Autodesk Inventor part; units mm, degrees
ref_plane "Work Plane1" through (0, 25, 0) normal (0, 1, 0) x (1, 0, 0)
ref_plane "Work Plane2" through (0, 0, 65) normal (0, 0, -1) x (-1, 0, 0)
ref_plane "YZ Plane" through (0, 0, 0) normal (1, 0, 0) x (0, 1, 0)
sketch "Sketch1" plane through (0, 0, 0) normal (0, 1, 0) x (-1, 0, 0)
  line L0 (0, 0) -> (100, 0)
  line L1 (100, 0) -> (100, 130)
  line L2 (100, 130) -> (0, 130)
  line L3 (0, 130) -> (0, 0)
  dimension "d0" = 130
  dimension "d1" = 100
extrude "Extrusion1" add sketch "Sketch1" along normal blind 50
sketch "Sketch2" plane through (0, 50, 0) normal (0, 1, 0) x (1, 0, 0)
  line L0 (-47, -106) -> (-10, -106)
  line L1 (-10, -106) -> (-10, -24)
  line L2 (-10, -24) -> (-47, -24)
  line L3 (-47, -24) -> (-47, -106)
  line L4 (0, -130) -> (0, 0)
  line L5 (-100, 0) -> (-100, -130)
  line L6 (-100, -130) -> (0, -130)
  line L7 (0, -130) -> (0, 0)
  line L8 (0, 0) -> (-100, 0)
  line L9 (-100, -65) -> (0, -65) construction
  point P0 (-47, -65)
  dimension "d4" = 82
  dimension "d5" = 37
  dimension "d6" = 10
extrude "Extrusion2" cut sketch "Sketch2" against normal blind 30 contours L3 L2 L1 L0
sketch "Sketch3" plane through (0, 0, 0) normal (0, -1, 0) x (1, 0, 0)
  line L0 (-96, 17.5) -> (-54, 17.5)
  line L1 (-54, 17.5) -> (-54, 112.5)
  line L2 (-54, 112.5) -> (-96, 112.5)
  line L3 (-96, 112.5) -> (-96, 17.5)
  line L4 (-100, 0) -> (-100, 130)
  line L5 (0, 0) -> (-100, 0)
  line L6 (0, 130) -> (0, 0)
  line L7 (-100, 130) -> (0, 130)
  line L8 (0, 65) -> (-100, 65) construction
  point P0 (-54, 65)
  dimension "d9" = 42
  dimension "d10" = 95
  dimension "d11" = 4
extrude "Extrusion3" cut sketch "Sketch3" against normal blind 27 contours L3 L2 L1 L0
ref_plane "Work Plane1" through (0, 25, 0) normal (0, 1, 0) x (1, 0, 0)
ref_plane "Work Plane2" through (0, 0, 65) normal (0, 0, -1) x (-1, 0, 0)
sketch "Sketch5" plane through (0, 0, 0) normal (0, 0, -1) x (-1, 0, 0)
  line L0 (0, 0) -> (100, 0)
  line L1 (100, 0) -> (100, 50)
  line L2 (0, 50) -> (100, 50)
  line L3 (0, 0) -> (0, 50)
  line L4 (-20, 25) -> (120, 25)
  arc A0 (0, 10) -> (0, 40) centre (0, 25) ccw
  arc A1 (48.5688, 34.5933) -> (11.5312, 34.5933) centre (30.05, 50) ccw
  arc A2 (11.5312, 15.4067) -> (48.5688, 15.4067) centre (30.05, 0) ccw
  circle A3 centre (60.1, 25) radius 15
  point P0 (54.1397, 50)
  point P1 (5.9603, 50)
  point P2 (5.9603, 0)
  point P3 (54.1397, 0)
  dimension "d14" = 30
  dimension "d15" = 60.1
extrude "Extrusion4" cut sketch "Sketch5" against normal blind 15 contours A2 A0 L4 A3 L0 | A0 A1 L2 A3 L4
mirror "Mirror1" about plane through (0, 0, 65) normal (0, 0, -1) of "Extrusion4"
sketch "Sketch6" plane through (0, 0, 15) normal (0, 0, -1) x (-1, 0, 0)
  arc A0 (48.5688, 34.5933) -> (54.1397, 50) centre (30.05, 50) ccw
  line L0 (5.9603, 50) -> (54.1397, 50)
  arc A1 (5.9603, 50) -> (11.5312, 34.5933) centre (30.05, 50) ccw
  arc A2 (11.5312, 15.4067) -> (11.5312, 34.5933) centre (0, 25) ccw
  arc A3 (11.5312, 15.4067) -> (5.9603, 0) centre (30.05, 0) ccw
  line L1 (54.1397, 0) -> (5.9603, 0)
  arc A4 (54.1397, 0) -> (48.5688, 15.4067) centre (30.05, 0) ccw
  arc A5 (48.5688, 34.5933) -> (48.5688, 15.4067) centre (60.1, 25) ccw
  arc A6 (24.9265, 50) -> (35.1735, 50) centre (30.05, 46) ccw
  arc A7 (35.1735, 0) -> (24.9265, 0) centre (30.05, 4) ccw
  line L2 (30.05, 50) -> (30.05, 0) construction
  line L3 (-20, 25) -> (120, 25)
  circle A8 centre (30.05, 4) radius 3.5
  circle A9 centre (30.05, 46) radius 3.5
  point P0 (0, 0)
  dimension "d18" = 13
  dimension "d19" = 42
  dimension "d20" = 21
  dimension "d21" = 7
extrude "Extrusion5" add sketch "Sketch6" along normal blind 5 contours A6 L0 | L1 A7
mirror "Mirror2" about plane through (0, 0, 65) normal (0, 0, -1) of "Extrusion5"
sketch "Sketch7" plane through (-100, 0, 0) normal (0, 0, -1) x (-1, 0, 0)
  circle A0 centre (-90, 25) radius 3
  circle A1 centre (-49.9, 25) radius 3
  arc A2 (-88.4688, 15.4067) -> (-94.0397, 0) centre (-69.95, 0) ccw
  arc A3 (-88.4688, 15.4067) -> (-88.4688, 34.5933) centre (-100, 25) ccw
  arc A4 (-94.0397, 50) -> (-88.4688, 34.5933) centre (-69.95, 50) ccw
  line L0 (-100, 50) -> (-94.0397, 50)
  line L1 (-100, 0) -> (-100, 50)
  line L2 (-100, 0) -> (-94.0397, 0)
  arc A5 (-45.8603, 0) -> (-51.4312, 15.4067) centre (-69.95, 0) ccw
  line L3 (-45.8603, 0) -> (0, 0)
  line L4 (0, 0) -> (0, 50)
  line L5 (-45.8603, 50) -> (0, 50)
  arc A6 (-51.4312, 34.5933) -> (-45.8603, 50) centre (-69.95, 50) ccw
  arc A7 (-51.4312, 34.5933) -> (-51.4312, 15.4067) centre (-39.9, 25) ccw
  line L6 (-120, 25) -> (20, 25)
  line L7 (-69.95, 0) -> (-69.95, 50) construction
  circle A8 centre (-29.8, 25) radius 3
  circle A9 centre (-15, 25) radius 3
  dimension "d24" = 6
  dimension "d25" = 6
  dimension "d26" = 40.1
  dimension "d27" = 20.05
  dimension "d30" = 20.1
  dimension "d31" = 14.8
extrude "Extrusion6" cut sketch "Sketch7" against normal blind 10 contours L6 A0 | A0 L6 | L6 A1 | A1 L6 | A8 L6 | L6 A8 | A9 L6 | L6 A9
mirror "Mirror3" about plane through (0, 0, 65) normal (0, 0, -1) of "Extrusion6"
equation "\"d20\" = 0.5 * d19"
equation "\"d27\" = 0.5 * d26"
properties part number "Full_Body"
Geometry check sheet. Reference: the model listing, model coordinates, mm. A direction names the side the tool comes from. Coordinates: 2 decimals unless noted, no trailing zeros. Order: outer loops, then holes, each group sorted by start corner. A loop starts at its lowest first (then second) coordinate and runs counter-clockwise, first axis right, second up. Notation, with made-up numbers: (46, 64) - (87, 64) arc R19 ccw to (87, 80) - close; hole circle Ø5 at (-19.75, 49.5). An arc over 180 degrees is marked (long way). Answer in a Markdown table with one row per item. Add a question column.
1. Section check B-B (x = -62). Enter the section's corners in (y, z).
2. Section check D-D (x = -21). Enter the section's corners in (y, z), plus the area to 3 significant figures.
3. Gauge pin test, flat ends, axial feed: pin 1 Ø3 at (x, z) = (-13, 60) entering from +Y; pin 2 Ø4 at (x, y) = (-36, 43.5) entering from -Z; pin 3 Ø5.5 at (x, y) = (-30.5, 4) entering from +Z. Record the tip position at first contact, or that the pin passes through.
4. Access from +Z, -Z, +X, -X, +Y, -Y to the whole of each face (thin tool, end or side, straight path). Record for faces 1 (the face through (-54, 13, 64)), 2 (the face through (-52.744, 41.919, 122.605)), 3 (the face through (-50, 25, 10)), 4 (the face through (-30, 8, 10)), 5 (the face through (-26.553, 4.154, 117.465)).
5. Draft check along Z on faces 6 (the face through (-29, 20, 64)), 7 (the face through (-30, 46, 115)), 8 (the face through (-30, 46, 15)), 9 (the face through (-29.59, 49.47, 117.46)). Enter one of: +Z half, -Z half, draft (parallel to the pull), parting line (faces both ways), or undercut.
6. Section check A-A (z = 13.5). Enter the section's corners in (x, y), plus the area to 3 significant figures.
7. Section check C-C (y = 30). Enter the section's corners in (x, z).
8. Material ranges on L1, parallel to X at y = 25, z = 128; L2, parallel to Y at x = -30, z = 13; L3, parallel to X at y = 25, z = 27.5, recorded low to high. Write a range as [from, to].
Data:
| question | item | result |
|---|---|---|
| 1 | outline | (0, 0) - (50, 0) - (50, 130) - (0, 130) - (0, 112.5) - (27, 112.5) - (27, 17.5) - (0, 17.5) - close |
| 2 | outline | (0, 15) - (50, 15) - (50, 24) - (20, 24) - (20, 106) - (50, 106) - (50, 115) - (0, 115) - close |
| 2 | area | 2,540 mm² |
| 3 | pin 1 | stops at y = 20 |
| 3 | pin 2 | stops at z = 10 |
| 3 | pin 3 | stops at z = 115 |
| 4 | face 1 | -Y |
| 4 | face 2 | +Z, +Y |
| 4 | face 3 | -Z |
| 4 | face 4 | -Z, +Y, -Y |
| 4 | face 5 | +Z |
| 5 | face 6 | undercut |
| 5 | face 7 | +Z half |
| 5 | face 8 | -Z half |
| 5 | face 9 | draft |
| 6 | outline | (-100, 0) - (-54.14, 0) arc R24.09 cw to (-48.57, 15.41) arc R15 ccw to (-48.57, 34.59) arc R24.09 cw to (-54.14, 50) - (-100, 50) - close; (-35.17, 0) - (-24.93, 0) arc R6.5 ccw (long way) to start; (-35.17, 50) arc R6.5 ccw (long way) to (-24.93, 50) - close; (-11.53, 15.41) arc R24.09 cw to (-5.96, 0) - (0, 0) - (0, 50) - (-5.96, 50) arc R24.09 cw to (-11.53, 34.59) arc R15 ccw to start; hole circle Ø7 at (-30.05, 4); hole circle Ø7 at (-30.05, 46) |
| 6 | area | 3,160 mm² |
| 7 | outline | (-100, 0) - (-45.96, 0) - (-45.96, 15) - (-14.14, 15) - (-14.14, 0) - (0, 0) - (0, 130) - (-14.14, 130) - (-14.14, 115) - (-45.96, 115) - (-45.96, 130) - (-100, 130) - close; hole (-47, 24) - (-10, 24) - (-10, 106) - (-47, 106) - close |
| 8 | L1 | x = [-100, -88], [-82, -73.2], [-67.2, -53.1], [-47.1, -45.1], [-15, -13], [-7, 0] |
| 8 | L2 | y = [0, 0.5], [7.5, 10.5], [39.5, 42.5], [49.5, 50] |
| 8 | L3 | x = [-100, -96], [-54, -47], [-10, 0] |
